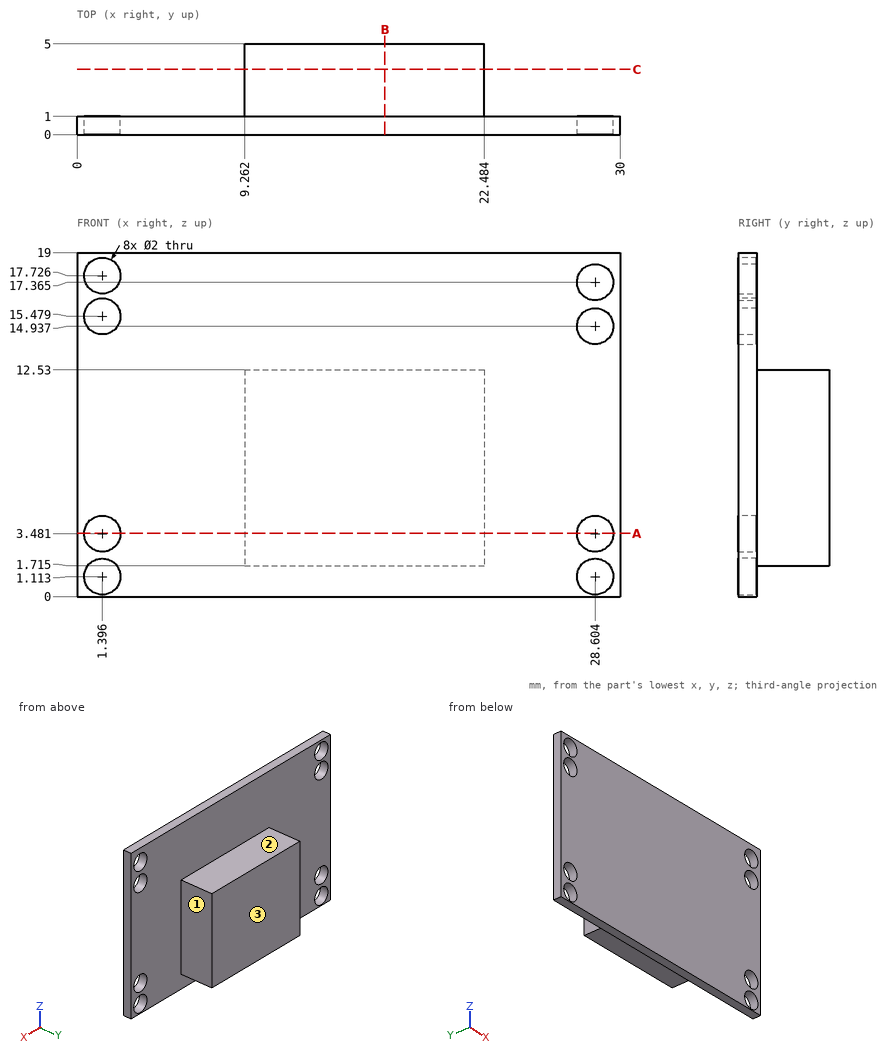
The figure shows three views and two pictorial views of one solid part (mm, origin at its lowest corner). Answer the questions. A direction names the side the tool comes from. Coordinates: 2 decimals unless noted, no trailing zeros. Loops run counter-clockwise (first coordinate to the right, second up) from the corner with the lowest first, then second, coordinate; pieces in that order, holes last. Notation, with made-up numbers: (48, 21) -> (85, 21) arc R21 cw to (85, 37) -> close; hole circle Ø10 at (70, 21.25). An arc over 180 degrees is marked (long way). Return JSON: item names as keys, results as strings. Group by question number.
(1) Given pin 1 Ø1.2 at (x, y) = (13.5, 3.5) entering from +Z; pin 2 Ø1.5 at (x, z) = (8, 6) entering from +Y; pin 3 Ø1 at (y, z) = (4.5, 8.5) entering from +X, each flat-ended and moving along its own axis, determine where each tip first touches the part or whether it passes through.
(2) Which of the six approach directions +Z, -Z, +X, -X, +Y, -Y give full straight-line access (tool end or side, diameter ignored) to the marked faces 1, 2 and 3?
(3) A cutting plane is placed at A-A on z = 3.5. Write down the section's boundary in (x, y).
(4) A cutting plane is placed at B-B on x = 17. Write down the section's boundary in (y, z) (1 decimal).
(5) A cutting plane is placed at C-C on y = 3.6. Write down the section's boundary in (x, z) (1 decimal), and give its area (3 significant figures).
(6) Find the intervals of material crossed by probe 1 along X at (y, z) = (0.7, 17.75) (1 decimal); probe 2 along Y at (x, z) = (3.75, 11.5); probe 3 along X at (y, z) = (0.5, 15.25) (1 decimal), in increasing order. Write a range as from..to.
The answers:
{
 "1": {"pin 1": "stops at z = 12.53", "pin 2": "stops at y = 1", "pin 3": "stops at x = 22.48"},
 "2": {"face 1": "+Z, -Z, +X, +Y", "face 2": "+Z, +X, -X, +Y", "face 3": "+Z, -Z, +X, -X, +Y"},
 "3": {"outline": "(0, 0) -> (0.4, 0) -> (0.4, 1) -> (0, 1) -> close; (2.4, 0) -> (27.6, 0) -> (27.6, 1) -> (22.48, 1) -> (22.48, 5) -> (9.26, 5) -> (9.26, 1) -> (2.4, 1) -> close; (29.6, 0) -> (30, 0) -> (30, 1) -> (29.6, 1) -> close"},
 "4": {"outline": "(0, 0) -> (1, 0) -> (1, 1.7) -> (5, 1.7) -> (5, 12.5) -> (1, 12.5) -> (1, 19) -> (0, 19) -> close"},
 "5": {"outline": "(9.3, 1.7) -> (22.5, 1.7) -> (22.5, 12.5) -> (9.3, 12.5) -> close", "area": "143 mm^2"},
 "6": {"probe 1": "x = 0..0.4, 2.4..27.7, 29.5..30", "probe 2": "y = 0..1", "probe 3": "x = 0..0.4, 2.4..27.7, 29.6..30"}
}
